For this review, use the dimensioned drawing (mm, ordinates from the lowest corner) and the shaded views. A direction names the side the tool comes from. Coordinates: 2 decimals unless noted, no trailing zeros. Loops run counter-clockwise (first coordinate to the right, second up) from the corner with the lowest first, then second, coordinate; pieces in that order, holes last. Notation, with made-up numbers: M 64.25,18 L 70.25,18 A10 cw 70.25,27 Z; hole C 7.25,20 d3. An arc over 180 degrees is marked long. One line per item, written item: value.
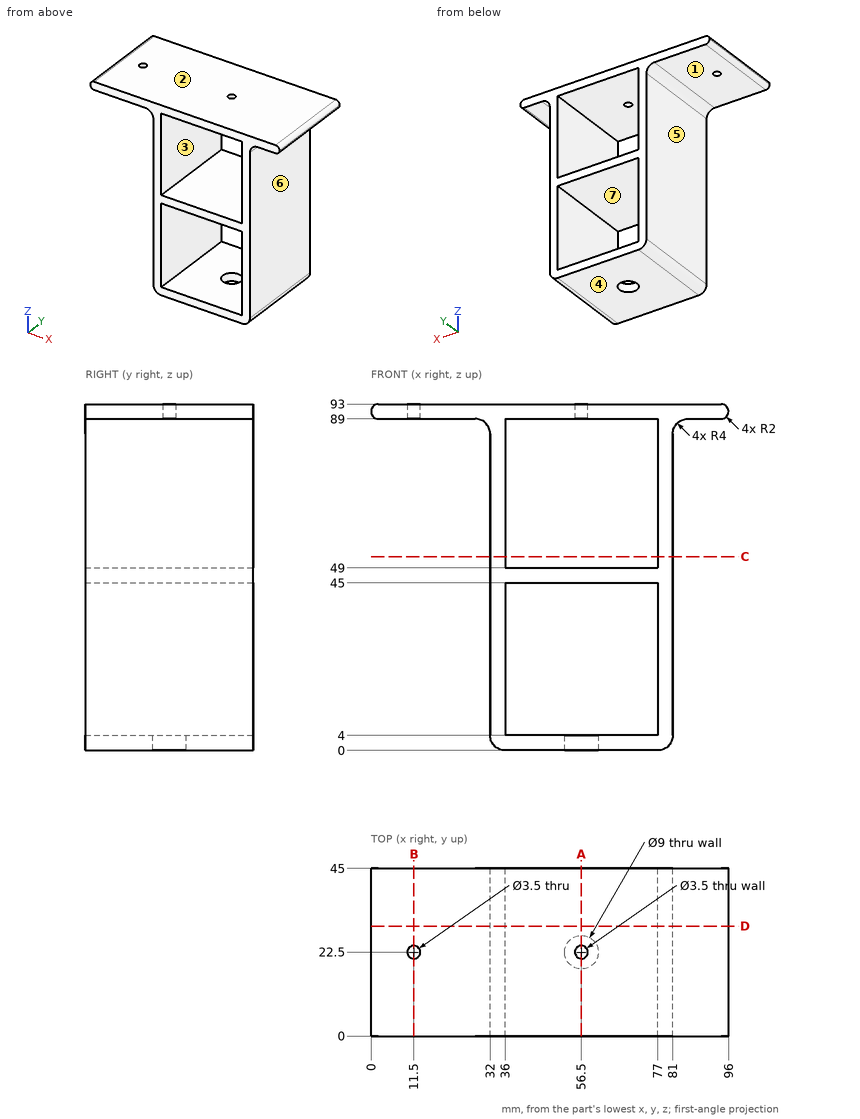
(1) Add section C-C on z = 52. State the section outline as (x, y) points.
Checks:
outline: M 32,0 L 36,0 L 36,45 L 32,45 Z; M 77,0 L 81,0 L 81,45 L 77,45 Z
(2) Tool access review of the marked faces 4, 5, 6 and 7: name each direction out of +Z, -Z, +X, -X, +Y, -Y from which nothing blocks a thin tool from reaching the whole face with its end or side.
Checks:
face 4: -Z, +X, -X, +Y, -Y
face 5: -Z, -X, +Y, -Y
face 6: -Z, +X, +Y, -Y
face 7: +Y, -Y
(3) Add section D-D on y = 29.5. State how many separate pieces and enclosed holes the cut face has, then the cut area to 3 significant figures.
Checks:
separate pieces: 1
enclosed holes: 2
area: 1,420 mm^2
(4) Insertion check: pin 1 Ø6 at (x, y) = (69.5, 38.5) entering from -Z; pin 2 Ø10 at (y, z) = (14, 31.5) entering from -X; pin 3 Ø21 at (x, y) = (18.5, 14) entering from -Z; pin 4 Ø2 at (x, y) = (56.5, 22.5) entering from -Z. Each pin has a flat end and moves straight along its axis. Give the tip position at first contact, or say it passes through.
Checks:
pin 1: z = 0
pin 2: x = 32
pin 3: z = 88.87
pin 4: z = 45
(5) To check wall thickness, follow L1, parallel to Z at x = 69, y = 35; L2, parallel to X at y = 5.5, z = 78; L3, parallel to X at y = 22, z = 91. State the ranges of each line that lie inside material, in increasing order. Write a range as [from, to].
Checks:
L1: [0, 4], [45, 49], [89, 93]
L2: [32, 36], [77, 81]
L3: [0, 9.82], [13.18, 54.82], [58.18, 96]
(6) Add section A-A on x = 56.5. State the section outline as (y, z) points.
Checks:
outline: M 0,0 L 18,0 L 18,4 L 0,4 Z; M 0,45 L 45,45 L 45,49 L 0,49 Z; M 0,89 L 20.75,89 L 20.75,93 L 0,93 Z; M 24.25,89 L 45,89 L 45,93 L 24.25,93 Z; M 27,0 L 45,0 L 45,4 L 27,4 Z
(7) Add section B-B on x = 11.5. State the section outline as (y, z) points, then the cut area to 3 significant figures.
Checks:
outline: M 0,89 L 20.75,89 L 20.75,93 L 0,93 Z; M 24.25,89 L 45,89 L 45,93 L 24.25,93 Z
area: 166 mm^2
(8) Draft analysis for pull direction Z (two halves, no side actions). For the marked faces 1, 2 and 3, state which applies: pulls with the +Z half, pulls with the -Z half, needs draft (parallel to the pull), parting line crosses it, or undercut.
Checks:
face 1: pulls with the -Z half
face 2: pulls with the +Z half
face 3: undercut
